```python
from build123d import *

# Parameters (mm, degrees)
SKETCH1_R           = 38.0746
SKETCH1_R_2         = 36.5125
BOSS_EXTRUDE1_DEPTH = 203.2
SKETCH2_R           = 3.175
CUT_EXTRUDE1_DEPTH  = 211.213202084
CIRPATTERN1_COUNT   = 4
SKETCH3_R           = 3.175
CUT_EXTRUDE2_DEPTH  = 297.323244266
CIRPATTERN2_COUNT   = 3


with BuildPart() as part:
    # Sketch1 → Boss-Extrude1 (new body)
    with BuildSketch(Plane.YZ):
        with Locations(Location((0, 0, 0), (0, 0, 270))):
            Circle(SKETCH1_R)
        with Locations(Location((0, 0, 0), (0, 0, 270))):
            Circle(SKETCH1_R_2, mode=Mode.SUBTRACT)
    extrude(amount=BOSS_EXTRUDE1_DEPTH)

    # Sketch2 → Cut-Extrude1 (cut, through all)
    with BuildSketch(Plane(origin=(0, 0, 0), x_dir=(-1, 0, 0), z_dir=(0, 1, 0))):
        with Locations(Location((-50.8, 0, 0), (0, 0, 270))):
            Circle(SKETCH2_R)
    cut_extrude1 = extrude(amount=CUT_EXTRUDE1_DEPTH, mode=Mode.SUBTRACT)

    # CirPattern1: Cut-Extrude1 ×4 about axis
    cirpattern1_axis = Axis((203.2, 0, 0), (-1, 0, 0))
    for i in range(1, CIRPATTERN1_COUNT):
        add(cut_extrude1.rotate(cirpattern1_axis, i * 360 / CIRPATTERN1_COUNT), mode=Mode.SUBTRACT)

    # Sketch3 → Cut-Extrude2 (cut, through all)
    with BuildSketch(Plane(origin=(0, 174.216591142, 0), x_dir=(-1, 0, 0), z_dir=(0, 0, 1))):
        with Locations((-152.4, 174.216591142)):
            Circle(SKETCH3_R)
    cut_extrude2 = extrude(amount=CUT_EXTRUDE2_DEPTH, mode=Mode.SUBTRACT)

    # CirPattern2: Cut-Extrude2 ×3 about axis
    cirpattern2_axis = Axis((203.2, 0, 0), (-1, 0, 0))
    for i in range(1, CIRPATTERN2_COUNT):
        add(cut_extrude2.rotate(cirpattern2_axis, i * 360 / CIRPATTERN2_COUNT), mode=Mode.SUBTRACT)


solid = part.part
```
The listing builds one solid part. Answer for the finished solid, in the listing's coordinates (mm). A direction names the side the tool comes from. Round coordinates to 2 decimals unless told otherwise and drop trailing zeros. Write each loop counter-clockwise with the first axis right and the second up, starting at its lowest first coordinate (ties: lowest second). Pieces come first, ordered by that corner, then holes. Notation, with made-up numbers: (-24.75, -11.5) -> (5.25, -11.5) arc R21 ccw to (5.25, 22.5) -> close; hole circle Ø11 at (84.25, -16). An arc over 180 degrees is marked (long way). Answer as a JSON object with one key per item and string values. Group by question number.
Q1. Section B-B (y = 0) is taken. Write down the section's boundary in (x, z) (1 decimal).
Q2. Section C-C (x = 152.4) is taken. Write down the section's boundary in (y, z) (1 decimal).
Q3. Section D-D (y = 17.5) is taken. Write down the section's boundary in (x, z).
Q4. Straight lines are drawn through the part: line 1 along X through (y, z) = (36.85, 0) (3 decimals); line 2 along Y through (x, z) = (182, -1.5); line 3 along Y through (x, z) = (68.5, 23). For each, find the intervals that lie inside material, in ascending order.
Q5. Determine the mould class of faces 3 (the face through (50.66, -3.17, 37.21)), 4 (the face through (203.2, -20, -31)), 5 (the face through (100.178, 11.437, -36.316)) for opening direction Y: pulls with the +Y half, pulls with the -Y half, needs draft (parallel to the pull), parting line crosses it, or undercut.
Q6. Section A-A (z = 0) is taken. Write down the section's boundary in (x, y) (1 decimal), plus the area to 3 significant figures.
Q7. Each of these flat-tipped pins is pushed along its axis until it touches: pin 1 Ø10 at (x, z) = (50.8, 0) entering from +Y; pin 2 Ø1.5 at (x, y) = (160, 1.5) entering from +Z; pin 3 Ø8 at (x, z) = (182, -18.5) entering from -Y; pin 4 Ø12 at (x, z) = (129.5, 21) entering from +Y. Where does it stop, or does it pass through?
Q8. Which of the six approach directions +Z, -Z, +X, -X, +Y, -Y give full straight-line access (tool end or side, diameter ignored) to faces 1 (the face through (150.693, -2.677, 37.213)), 2 (the face through (50.66, -37.21, -3.17))?
Check values:
{
 "1": {"outline": "(0, -38.1) -> (47.6, -38.1) -> (47.6, -36.5) -> (0, -36.5) -> close; (0, 36.5) -> (47.6, 36.5) -> (47.6, 38.1) -> (0, 38.1) -> close; (54, -38.1) -> (203.2, -38.1) -> (203.2, -36.5) -> (54, -36.5) -> close; (54, 36.5) -> (149.2, 36.5) -> (149.2, 38.1) -> (54, 38.1) -> close; (155.6, 36.5) -> (203.2, 36.5) -> (203.2, 38.1) -> (155.6, 38.1) -> close"},
 "2": {"outline": "(-34.4, -16.2) -> (-33.1, -15.4) arc R36.5 cw to (-3.2, 36.4) -> (-3.2, 37.9) arc R38.1 ccw to start; (-31.3, -21.7) arc R38.1 ccw to (31.3, -21.7) -> (29.9, -20.9) arc R36.5 cw to (-29.9, -20.9) -> close; (3.2, 36.4) arc R36.5 cw to (33.1, -15.4) -> (34.4, -16.2) arc R38.1 ccw to (3.2, 37.9) -> close"},
 "3": {"outline": "(0, -33.81) -> (203.2, -33.81) -> (203.2, -32.05) -> (0, -32.05) -> close; (0, 32.05) -> (203.2, 32.05) -> (203.2, 33.81) -> (0, 33.81) -> close"},
 "4": {"line 1": "0 to 47.625, 53.975 to 203.2", "line 2": "-38.05 to -36.48, 36.48 to 38.05", "line 3": "-30.34 to -28.36, 28.36 to 30.34"},
 "5": {"face 3": "undercut", "face 4": "needs draft", "face 5": "parting line crosses it"},
 "6": {"outline": "(0, -38.1) -> (47.6, -38.1) -> (47.6, -36.5) -> (0, -36.5) -> close; (0, 36.5) -> (47.6, 36.5) -> (47.6, 38.1) -> (0, 38.1) -> close; (54, -38.1) -> (203.2, -38.1) -> (203.2, -36.5) -> (54, -36.5) -> close; (54, 36.5) -> (203.2, 36.5) -> (203.2, 38.1) -> (54, 38.1) -> close", "area": "615 mm^2"},
 "7": {"pin 1": "y = 38.07", "pin 2": "z = 38.07", "pin 3": "y = -35.21", "pin 4": "y = 35"},
 "8": {"face 1": "+Z", "face 2": "+Y, -Y"}
}
